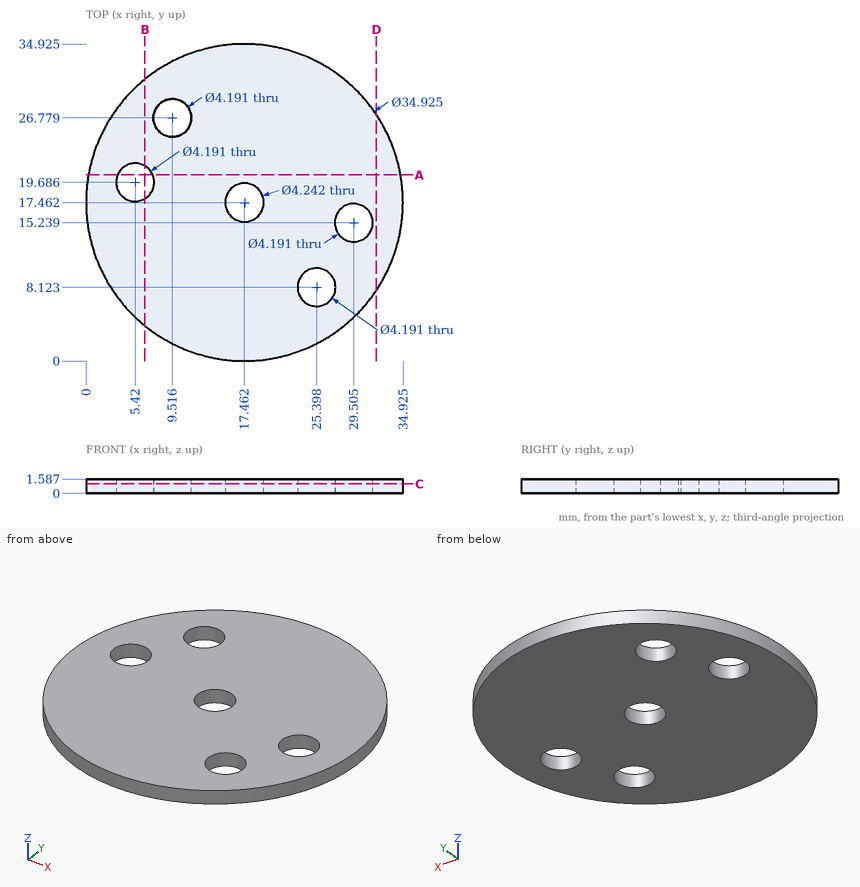
The drawing under review shows one solid part. Ordinate dimensions are in mm from its lowest x, y, z. Round coordinates to 2 decimals unless told otherwise and drop trailing zeros. Write each loop counter-clockwise with the first axis right and the second up, starting at its lowest first coordinate (ties: lowest second). Pieces come first, ordered by that corner, then holes. Notation, with made-up numbers: M 60.25,24.25 L 81.25,24.25 A28 cw 81.25,63.25 Z; hole C -24.5,11 d2. An arc over 180 degrees is marked long. One line per item, written item: value. Start each with the question number.
(1) Insertion check: pin 1 (8 mm diameter, centred on x = 6.5, y = 17.5, fed in from -Z); pin 2 (2.5 mm diameter, centred on x = 29.5, y = 15.24, fed in from -Z). Each pin has a flat end and moves straight along its axis. Give the tip position at first contact, or say it passes through.
(2) Wall thickness on line 1 (X direction, y = 19, z = 0.5) (1 decimal); line 2 (X direction, y = 13.5, z = 1.3) (1 decimal); line 3 (Y direction, x = 7, z = 1.1) (1 decimal): over which ranges is each line inside the solid? List them lowest first.
(3) We need section C-C (z = 1.05). Give the boundary of the cut face in (x, y) (1 decimal).
(4) We need section A-A (y = 20.5). Give the boundary of the cut face in (x, z).
(5) We need section B-B (x = 6.5). Give the boundary of the cut face in (y, z) (1 decimal).
(6) We need section D-D (x = 32). Give the boundary of the cut face in (y, z).
Result:
1. pin 1: z = 0
1. pin 2: through
2. line 1: 0.1 to 3.4, 7.4 to 16, 18.9 to 34.9
2. line 2: 0.5 to 28.3, 30.7 to 34.5
2. line 3: 3.5 to 18.3, 21.1 to 31.4
3. outline: C 17.5,17.5 d34.9; hole C 5.4,19.7 d4.2; hole C 9.5,26.8 d4.2; hole C 17.5,17.5 d4.2; hole C 25.4,8.1 d4.2; hole C 29.5,15.2 d4.2
4. outline: M 0.27,0 L 3.49,0 L 3.49,1.59 L 0.27,1.59 Z; M 7.35,0 L 34.66,0 L 34.66,1.59 L 7.35,1.59 Z
5. outline: M 3.9,0 L 17.9,0 L 17.9,1.6 L 3.9,1.6 Z; M 21.5,0 L 31.1,0 L 31.1,1.6 L 21.5,1.6 Z
6. outline: M 7.79,0 L 27.14,0 L 27.14,1.59 L 7.79,1.59 Z
